Verification items for the finished model (mm, model axes). Face numbers are marked on the shaded views. A direction names the side the tool comes from. Give positions to 0.01 mm unless a question says otherwise; leave off trailing zeros. Order: outer loops, then holes, each group sorted by start corner. A loop starts at its lowest first (then second) coordinate and runs counter-clockwise, first axis right, second up.
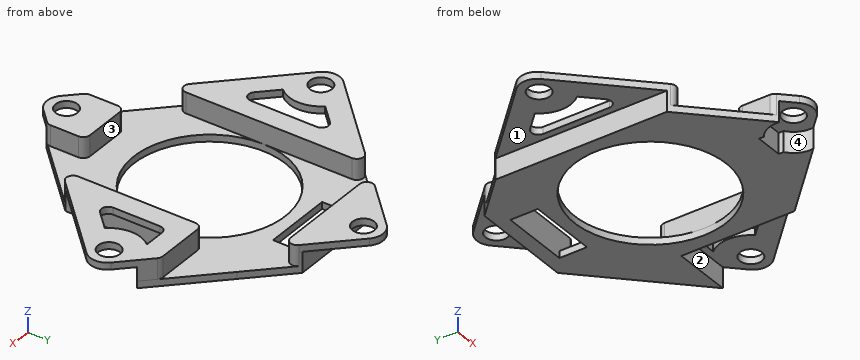
from build123d import *

# Parameters (mm, degrees)
F0_R         = 1.6
F1_DEPTH     = 1
F2_ANGLE     = 45
F3_DEPTH     = 4
F5_DEPTH     = 3
F20_DEPTH    = 3
F7_R         = 11
F8_DEPTH     = 25
F9_DEPTH     = 3
F10_W        = 10
F10_H        = 4
F11_DEPTH    = 25
F13_DEPTH    = 25
F14_DEPTH    = 1
F15_DEPTH    = 2
F16_DEPTH    = 1
F17_DEPTH    = 2
F18_T1_DEPTH = 5.5
F18_T3_DEPTH = 9.0355339059
F18_T5_DEPTH = 4.0355339059


# Not quite as in the source:
# - a fillet or chamfer that OpenCascade refuses, or shapes differently, is made with other operations: its cross-section is extruded or revolved along the edge and cut away or added


with BuildPart() as f1:
    # F0 (on Top) → F1 (new body)
    with BuildSketch(Plane.XY):
        with BuildLine():
            Line((-14.7650561035, -22.9090262799), (16.2349438965, -22.9090262799))
            ThreePointArc((16.2349438965, -22.9090262799), (18.0027108495, -22.1767932329), (18.7349438965, -20.4090262799))
            Line((18.7349438965, -20.4090262799), (18.7349438965, 10.5909737201))
            ThreePointArc((18.7349438965, 10.5909737201), (18.0027108495, 12.3587406731), (16.2349438965, 13.0909737201))
            Line((16.2349438965, 13.0909737201), (-14.7650561035, 13.0909737201))
            ThreePointArc((-14.7650561035, 13.0909737201), (-16.5328230564, 12.3587406731), (-17.2650561035, 10.5909737201))
            Line((-17.2650561035, 10.5909737201), (-17.2650561035, -20.4090262799))
            ThreePointArc((-17.2650561035, -20.4090262799), (-16.5328230564, -22.1767932329), (-14.7650561035, -22.9090262799))
        make_face()
        with Locations((-14.5150561035, -20.1590262799)):
            Circle(F0_R, mode=Mode.SUBTRACT)
        with Locations((15.9849438965, -20.1590262799)):
            Circle(F0_R, mode=Mode.SUBTRACT)
        with Locations((-14.5150561035, 10.3409737201)):
            Circle(F0_R, mode=Mode.SUBTRACT)
        with Locations((15.9849438965, 10.3409737201)):
            Circle(F0_R, mode=Mode.SUBTRACT)
    extrude(amount=F1_DEPTH)


with BuildPart() as f1_1:
    # F2: moved
    add(f1.part.rotate(Axis((16.2349438965, -22.9090262799, 0.5), (0, 0, -1)), F2_ANGLE))

    # F19 (on face) → F3 (join)
    with BuildSketch(Plane.XY.offset(1)):
        Polygon((10.5468667268, -17.2209491102), (25.4585549722, -17.2209491102), (31.0027108495, -11.6767932329), (31.0027108495, 13.2348950126), (25.4585549722, 18.7790508898), (10.5468667268, 18.7790508898), (5.0027108495, 13.2348950126), (5.0027108495, -11.6767932329), align=None)
    extrude(amount=-F3_DEPTH)

    # F4 (on face) → F5 (cut)
    with BuildSketch(Plane.XY.offset(1)):
        Polygon((8.5468667268, -15.2209491102), (27.4585549722, -15.2209491102), (29.0027108495, -13.6767932329), (29.0027108495, 15.2348950126), (27.4585549722, 16.7790508898), (8.5468667268, 16.7790508898), (7.0027108495, 15.2348950126), (7.0027108495, -13.6767932329), align=None)
    extrude(amount=-F5_DEPTH, mode=Mode.SUBTRACT)

    # F6 (on face) → F20 (cut, through all)
    with BuildSketch(Plane.XY.offset(1)):
        Polygon((14.0027108495, -20.6767932329), (14.0027108495, -15.2209491102), (8.5468667268, -15.2209491102), align=None)
        Polygon((27.4585549722, -15.2209491102), (22.0027108495, -15.2209491102), (22.0027108495, -20.6767932329), align=None)
    extrude(amount=-F20_DEPTH, mode=Mode.SUBTRACT)

    # F7 (on face) → F8 (cut)
    with BuildSketch(Plane(origin=(0, 0, -3), x_dir=(1, 0, 0), z_dir=(0, 0, -1))):
        with Locations((18.0027108495, 0)):
            Circle(F7_R)
    extrude(amount=-F8_DEPTH, mode=Mode.SUBTRACT)

    # F21 (on face) → F9 (cut, through all)
    with BuildSketch(Plane.XY.offset(1)):
        Polygon((29.0027108495, 15.2348950126), (29.0027108495, 6.7790508898), (37.4585549722, 6.7790508898), align=None)
    extrude(amount=-F9_DEPTH, mode=Mode.SUBTRACT)

    # F10 (on face) → F11 (cut)
    with BuildSketch(Plane.XY.offset(-2)):
        with Locations((18.0027108495, 14.7790508898)):
            Rectangle(F10_W, F10_H)
    extrude(amount=-F11_DEPTH, mode=Mode.SUBTRACT)

    # F12 (on face) + F22 (on face) → F13 (cut)
    with BuildSketch(Plane.XY.offset(1)):
        with BuildLine():
            ThreePointArc((36.1448070539, -2.2920563414), (34.9697110872, 0.7317293655), (36.0823485209, 3.7790508898))
            Line((36.0823485209, 3.7790508898), (33.0027108495, 3.7790508898))
            ThreePointArc((33.0027108495, 3.7790508898), (32.2956040683, 3.486157671), (32.0027108495, 2.7790508898))
            Line((32.0027108495, 2.7790508898), (32.0027108495, -4.0199389834))
            ThreePointArc((32.0027108495, -4.0199389834), (32.6200274171, -4.9438185159), (33.7098176307, -4.7270457646))
            Line((33.7098176307, -4.7270457646), (36.1448070539, -2.2920563414))
        make_face()
    with BuildSketch(Plane.XY.offset(1)):
        with BuildLine():
            ThreePointArc((-0.1393853549, 3.8501581211), (1.0359540233, 0.7790508898), (-0.1393853549, -2.2920563414))
            Line((-0.1393853549, -2.2920563414), (2.2956040683, -4.7270457646))
            ThreePointArc((2.2956040683, -4.7270457646), (3.3853942819, -4.9438185159), (4.0027108495, -4.0199389834))
            Line((4.0027108495, -4.0199389834), (4.0027108495, 5.5780407631))
            ThreePointArc((4.0027108495, 5.5780407631), (3.3853942819, 6.5019202956), (2.2956040683, 6.2851475443))
            Line((2.2956040683, 6.2851475443), (-0.1393853549, 3.8501581211))
        make_face()
    extrude(amount=-F13_DEPTH, mode=Mode.SUBTRACT)

    # F23 (on face) → F14 (join, through all)
    with BuildSketch(Plane(origin=(0, 0, -3), x_dir=(1, 0, 0), z_dir=(0, 0, -1))):
        with BuildLine():
            Line((14.527236112, 21.2013184954), (10.5468667268, 17.2209491102))
            Line((10.5468667268, 17.2209491102), (16.0027108495, 17.2209491102))
            Line((16.0027108495, 17.2209491102), (16.0027108495, 17.9154246131))
            ThreePointArc((16.0027108495, 17.9154246131), (14.809831185, 19.3539976507), (14.527236112, 21.2013184954))
        make_face()
        with BuildLine():
            Line((20.0027108495, 17.9154246131), (20.0027108495, 17.2209491102))
            Line((20.0027108495, 17.2209491102), (25.4585549722, 17.2209491102))
            Line((25.4585549722, 17.2209491102), (21.478185587, 21.2013184954))
            ThreePointArc((21.478185587, 21.2013184954), (21.195590514, 19.3539976507), (20.0027108495, 17.9154246131))
        make_face()
    extrude(amount=-F14_DEPTH)

    # F24 (on face) → F15 (join, through all)
    with BuildSketch(Plane.XY.offset(-2)):
        with BuildLine():
            Line((22.0027108495, -20.6767932329), (22.0027108495, -17.2209491102))
            Line((22.0027108495, -17.2209491102), (20.0027108495, -17.2209491102))
            Line((20.0027108495, -17.2209491102), (20.0027108495, -17.9154246131))
            ThreePointArc((20.0027108495, -17.9154246131), (21.195590514, -19.3539976507), (21.478185587, -21.2013184954))
            Line((21.478185587, -21.2013184954), (22.0027108495, -20.6767932329))
        make_face()
        with BuildLine():
            Line((16.0027108495, -17.2209491102), (14.0027108495, -17.2209491102))
            Line((14.0027108495, -17.2209491102), (14.0027108495, -20.6767932329))
            Line((14.0027108495, -20.6767932329), (14.527236112, -21.2013184954))
            ThreePointArc((14.527236112, -21.2013184954), (14.809831185, -19.3539976507), (16.0027108495, -17.9154246131))
            Line((16.0027108495, -17.9154246131), (16.0027108495, -17.2209491102))
        make_face()
    extrude(amount=F15_DEPTH)

    # F25 (on face) → F16 (join, through all)
    with BuildSketch(Plane(origin=(0, 0, -3), x_dir=(1, 0, 0), z_dir=(0, 0, -1))):
        Polygon((31.0027108495, -4.7790508898), (31.0027108495, -13.2348950126), (39.4585549722, -4.7790508898), align=None)
    extrude(amount=-F16_DEPTH)

    # F26 (on face) → F17 (join, through all)
    with BuildSketch(Plane.XY.offset(-2)):
        Polygon((37.4585549722, 6.7790508898), (31.0027108495, 6.7790508898), (31.0027108495, 4.7790508898), (39.4585549722, 4.7790508898), align=None)
    extrude(amount=F17_DEPTH)

    # F18: fillet of radius 1 on 11 edges, made by hand

    # F18_s2 → F18_t1 (cut)
    with BuildSketch(Plane.XY.offset(-2)):
        with BuildLine():
            ThreePointArc((22.0027108495, -16.2209491102), (21.7098176307, -15.513842329), (21.0027108495, -15.2209491102))
            Line((21.0027108495, -15.2209491102), (22.0027108495, -15.2209491102))
            Line((22.0027108495, -15.2209491102), (22.0027108495, -16.2209491102))
        make_face()
        with BuildLine():
            ThreePointArc((15.0027108495, -15.2209491102), (14.2956040683, -15.513842329), (14.0027108495, -16.2209491102))
            Line((14.0027108495, -16.2209491102), (14.0027108495, -15.2209491102))
            Line((14.0027108495, -15.2209491102), (15.0027108495, -15.2209491102))
        make_face()
        with BuildLine():
            ThreePointArc((30.0027108495, 6.7790508898), (29.2956040683, 6.486157671), (29.0027108495, 5.7790508898))
            Line((29.0027108495, 5.7790508898), (29.0027108495, 6.7790508898))
            Line((29.0027108495, 6.7790508898), (30.0027108495, 6.7790508898))
        make_face()
    extrude(amount=F18_T1_DEPTH, mode=Mode.SUBTRACT)

    # F18_s4 → F18_t3 (cut)
    with BuildSketch(Plane.XY.offset(-2)):
        with BuildLine():
            ThreePointArc((5.2956040683, -11.9696864517), (6.3853942819, -12.186459203), (7.0027108495, -11.2625796705))
            Line((7.0027108495, -11.2625796705), (7.0027108495, -13.6767932329))
            Line((7.0027108495, -13.6767932329), (5.2956040683, -11.9696864517))
        make_face()
        with BuildLine():
            ThreePointArc((5.2956040683, 13.5277882314), (6.3853942819, 13.7445609827), (7.0027108495, 12.8206814502))
            Line((7.0027108495, 12.8206814502), (7.0027108495, 15.2348950126))
            Line((7.0027108495, 15.2348950126), (5.2956040683, 13.5277882314))
        make_face()
        with BuildLine():
            ThreePointArc((29.0027108495, -11.2625796705), (29.6200274171, -12.186459203), (30.7098176307, -11.9696864517))
            Line((30.7098176307, -11.9696864517), (29.0027108495, -13.6767932329))
            Line((29.0027108495, -13.6767932329), (29.0027108495, -11.2625796705))
        make_face()
        with BuildLine():
            ThreePointArc((10.253973508, 18.486157671), (10.0372007566, 17.3963674575), (10.9610802892, 16.7790508898))
            Line((10.9610802892, 16.7790508898), (8.5468667268, 16.7790508898))
            Line((8.5468667268, 16.7790508898), (10.253973508, 18.486157671))
        make_face()
        with BuildLine():
            ThreePointArc((25.751448191, 18.486157671), (25.9682209424, 17.3963674575), (25.0443414098, 16.7790508898))
            Line((25.0443414098, 16.7790508898), (27.4585549722, 16.7790508898))
            Line((27.4585549722, 16.7790508898), (25.751448191, 18.486157671))
        make_face()
    extrude(amount=F18_T3_DEPTH, mode=Mode.SUBTRACT)

    # F18_s6 → F18_t5 (cut)
    with BuildSketch(Plane.XY.offset(-2)):
        with BuildLine():
            ThreePointArc((14.2956040683, -20.9696864517), (14.078831317, -20.6452631029), (14.0027108495, -20.2625796705))
            Line((14.0027108495, -20.2625796705), (14.0027108495, -20.6767932329))
            Line((14.0027108495, -20.6767932329), (14.2956040683, -20.9696864517))
        make_face()
        with BuildLine():
            ThreePointArc((21.7098176307, -20.9696864517), (21.926590382, -20.6452631029), (22.0027108495, -20.2625796705))
            Line((22.0027108495, -20.2625796705), (22.0027108495, -20.6767932329))
            Line((22.0027108495, -20.6767932329), (21.7098176307, -20.9696864517))
        make_face()
        with BuildLine():
            ThreePointArc((37.751448191, 6.486157671), (37.4270248422, 6.7029304224), (37.0443414098, 6.7790508898))
            Line((37.0443414098, 6.7790508898), (37.4585549722, 6.7790508898))
            Line((37.4585549722, 6.7790508898), (37.751448191, 6.486157671))
        make_face()
    extrude(amount=F18_T5_DEPTH, mode=Mode.SUBTRACT)


solid = f1_1.part
(1) Section check A-A, the plane y = -3. Enter the section's corners in (x, z).
Solved:
outline: (-3.67, 0) - (0.57, 0) - (0.57, 1) - (-3.67, 1) - close; (4, 0) - (5, 0) - (5, -3) - (7.42, -3) - (7.42, -2) - (7, -2) - (7, 1) - (4, 1) - close; (28.59, -3) - (31, -3) - (31, 0) - (32, 0) - (32, 1) - (29, 1) - (29, -2) - (28.59, -2) - close; (35.44, 0) - (39.68, 0) - (39.68, 1) - (35.44, 1) - close
(2) Set-up check for the marked faces 1, 2, 3 and 4: record each of +Z, -Z, +X, -X, +Y, -Y from which the full face is reachable in a straight line by a thin tool's end or side.
Solved:
face 1: -Z, -X, +Y, -Y
face 2: -Z, +X, -Y
face 3: +Z, +X, -X
face 4: -Z
(3) Section check B-B, the plane x = 3. Enter the section's corners in (y, z), then the cut area to 3 significant figures.
Solved:
outline: (-9.67, 0) - (-5.02, 0) - (-5.02, 1) - (-9.67, 1) - close; (6.58, 0) - (11.23, 0) - (11.23, 1) - (6.58, 1) - close
area: 9.31 mm2
(4) Scan lines: line 1 (X direction, y = -1.5, z = 0.2); line 2 (X direction, y = 5, z = 0.3); line 3 (X direction, y = -0.5, z = -1.2). Record each from-to range of solid material in increasing order.
Solved:
line 1: x = -5.17 to 0.43, 4 to 7, 29 to 32, 35.57 to 41.18
line 2: x = -3.23 to 1.01, 4 to 7, 29 to 39.24
line 3: x = 5 to 7, 29 to 31
(5) Go/stop test with flat-tipped pins: pin 1 (12.5 mm diameter, centred on x = -2, y = -4, fed in from -Z); pin 2 (0.8 mm diameter, centred on x = 34, z = 0.5, fed in from -Y); pin 3 (20 mm diameter, centred on x = 18, y = 0, fed in from +Z); pin 4 (8 mm diameter, centred on x = 18.5, y = 11.5, fed in from +Z). Record where each tip stops, or that it passes through.
Solved:
pin 1: stops at z = 0
pin 2: stops at y = -9.08
pin 3: passes through
pin 4: stops at z = -2
